```python
from build123d import *

# Parameters (mm, degrees)
BOSS_EXTRUDE1_DEPTH = 12.7


with BuildPart() as part:
    # Sketch1 → Boss-Extrude1 (new body)
    with BuildSketch(Plane(origin=(0, 0, 0), x_dir=(1, 0, 0), z_dir=(0, 1, 0))):
        with BuildLine():
            Line((-38.1, -173.409838579), (-38.1, -148.009838579))
            Line((-38.1, -148.009838579), (0, -148.009838579))
            Line((0, -148.009838579), (0, -177.546))
            ThreePointArc((0, -177.546), (-19.161927299, -176.508930817), (-38.1, -173.409838579))
        make_face()
    boss_extrude1 = extrude(amount=BOSS_EXTRUDE1_DEPTH)

    # Mirror1: Boss-Extrude1 across plane
    add(boss_extrude1.mirror(Plane(origin=(0, 12.7, 148.009838579), x_dir=(0, 0, 1), z_dir=(-1, 0, 0))))


solid = part.part
```
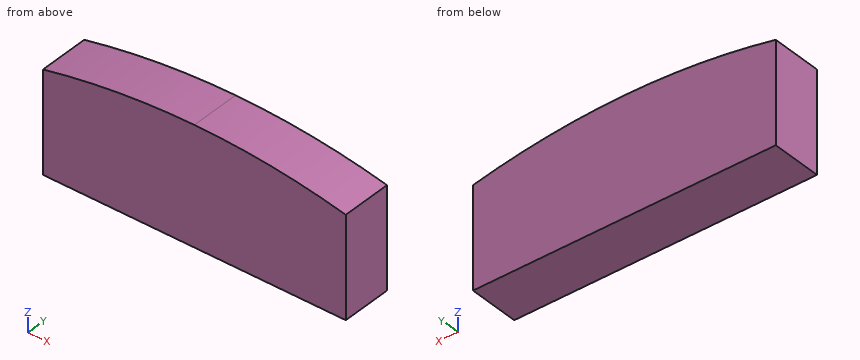
Could you check a few things on this model? Use its own coordinates, in mm. Give positions to 0.01 mm unless a question says otherwise; leave off trailing zeros. Loops run counter-clockwise (first coordinate to the right, second up) from the corner with the lowest first, then second, coordinate; pieces in that order, holes last. Notation, with made-up numbers: (87, 41.5) - (97, 41.5) arc R19 cw to (97, 50.5) - close; hole circle Ø7 at (-21, -38.75). An arc over 180 degrees is marked (long way). Answer in a Markdown table with one row per item. Add a question column.
Q1. If we section it at A-A (y = 8.5): List the corners of the cut face in (x, z) for me, plus the area to 3 significant figures.
Q2. Please list where these lines run through material, in increasing order: L1, parallel to Z at x = 23.5, y = 4; L2, parallel to Z at x = 6, y = 8.5. Write a range as from..to.
Q3. For pin 1 (1 mm diameter, centred on x = 22.5, z = 170.5, fed in from -Y); pin 2 (3 mm diameter, centred on x = -11, y = 11, fed in from +Z); pin 3 (3 mm diameter, centred on x = 29.5, y = 2.5, fed in from +Z), each with a flat end and sliding along its axis, tell me the tip position at first contact or that it passes through.
Q4. If we section it at C-C (x = 32): List the corners of the cut face in (y, z) for me.
Q5. If we section it at B-B (x = 20): List the corners of the cut face in (y, z) for me.
The answers:
| question | item | result |
|---|---|---|
| 1 | outline | (-38.1, 148.01) - (38.1, 148.01) - (38.1, 173.41) arc R177.55 ccw to (-38.1, 173.41) - close |
| 1 | area | 2,150 mm^2 |
| 2 | L1 | z = 148.01..175.98 |
| 2 | L2 | z = 148.01..177.44 |
| 3 | pin 1 | stops at y = 0 |
| 3 | pin 2 | stops at z = 177.29 |
| 3 | pin 3 | stops at z = 175.32 |
| 4 | outline | (0, 148.01) - (12.7, 148.01) - (12.7, 174.64) - (0, 174.64) - close |
| 5 | outline | (0, 148.01) - (12.7, 148.01) - (12.7, 176.42) - (0, 176.42) - close |
